Geometry: see drawing. Coordinates: mm, zero at the bounding-box minimum. A direction names the side the tool comes from. Coordinates: 2 decimals unless noted, no trailing zeros. Write each loop counter-clockwise with the first axis right and the second up, starting at its lowest first coordinate (ties: lowest second). Pieces come first, ordered by that corner, then holes. Notation, with made-up numbers: M 84,78 L 143,78 A18 cw 143,101 Z; hole C 51,49 d11. An arc over 180 degrees is marked long. One line per item, written item: value. Start each with the question number.
Item 1: Cut plane B-B, the plane z = 12. Output: boundary loops of the cut face in (x, y), then the cut area to 3 significant figures.
Item 2: Ray query, L1, parallel to X at y = 24, z = 17.75 (1 decimal); L2, parallel to Z at x = 5, y = 15; L3, parallel to Y at x = 23.81, z = 2.3. Return the intervals inside material, ascending. Write a range as from..to.
Item 3: Cut plane A-A, the plane x = 7.5. Output: boundary loops of the cut face in (y, z) (1 decimal).
Item 4: Mould query, pull axis X, two halves, no side actions, for the marked faces 1, 2, 3 and 4. Classes: released by +X, released by -X, zero draft, split by the parting line, or undercut.
Item 5: Cut plane C-C, the plane y = 4.5. Output: boundary loops of the cut face in (x, z).
Item 6: Pin query (flat end, axial travel): P1, Ø1.6, axis at x = 34.49, y = 35.25, coming from the -Z side; P2, Ø4, axis at y = 24.5, z = 20, coming from the +X side; P3, Ø1, axis at x = 27.5, y = 9.5, coming from the +Z side; P4, Ø2.5, axis at x = 23, y = 25.5, coming from the -Z side. Return the tip coordinate at first contact, or that it passes through.
Item 7: Set-up query: the marked faces 5 and 6. Return all of +Z, -Z, +X, -X, +Y, -Y with unobstructed straight access to the full face (end or side cutting, diameter ignored); none if empty.
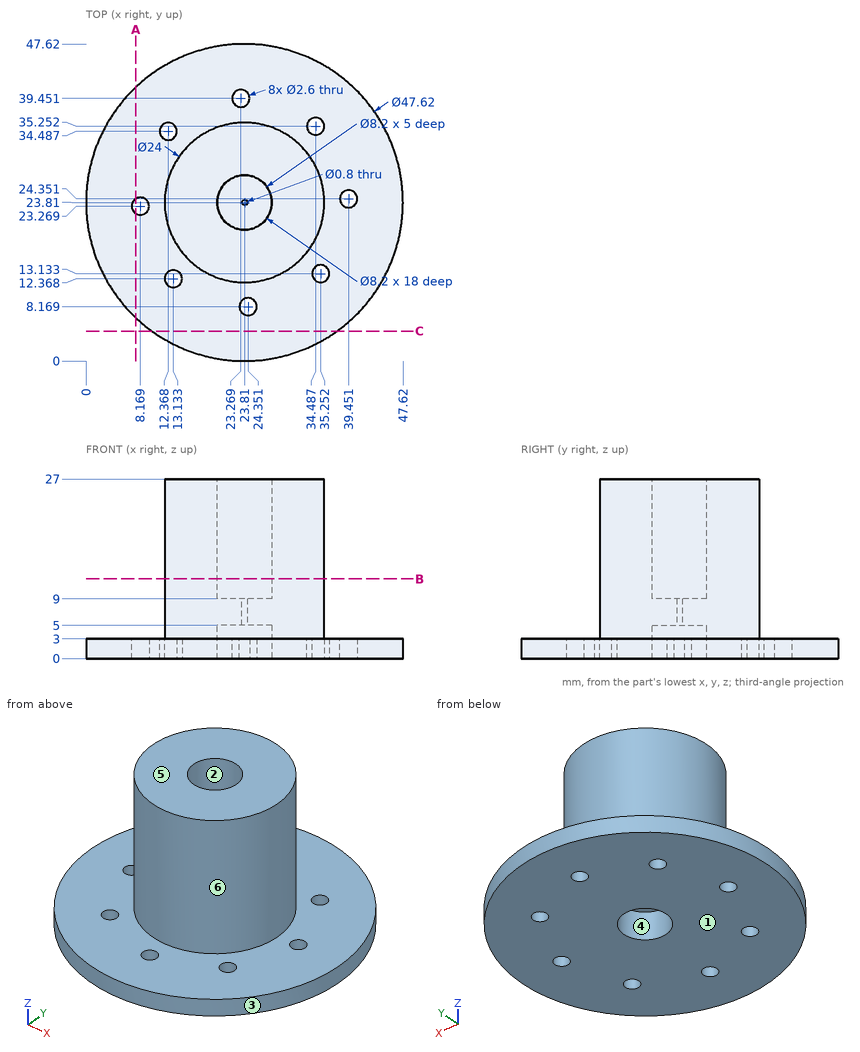
From the geometry:
1. outline: C 23.81,23.81 d24; hole C 23.81,23.81 d8.2
1. area: 400 mm²
2. L1: x = 11.8..19.7, 27.9..35.8
2. L2: z = 0..3
2. L3: y = 0..6.99, 9.35..19.71, 27.91..38.27, 40.63..47.62
3. outline: M 6.5,0 L 22.2,0 L 22.2,3 L 6.5,3 Z; M 24.4,0 L 41.2,0 L 41.2,3 L 24.4,3 Z
4. face 1: zero draft
4. face 2: undercut
4. face 3: split by the parting line
4. face 4: undercut
5. outline: M 9.88,0 L 37.74,0 L 37.74,3 L 9.88,3 Z
6. P1: passes through
6. P2: stops at x = 35.81
6. P3: stops at z = 3
6. P4: stops at z = 5
7. face 5: +Z, +X, -X, +Y, -Y
7. face 6: +Z
